from build123d import *

# Parameters (mm, degrees)
SKETCH2_R               = 12.5
BOSS_EXTRUDE1_DEPTH     = 20
CUT_EXTRUDE1_DEPTH      = 13.5
CUT_EXTRUDE1_DEPTH_BACK = 13.5
SKETCH4_R               = 3
CUT_EXTRUDE2_DEPTH      = 3


with BuildPart() as part:
    # Sketch2 → Boss-Extrude1 (new body, symmetric)
    with BuildSketch(Plane(origin=(0, 0, 0), x_dir=(1, 0, 0), z_dir=(0, 1, 0))):
        Circle(SKETCH2_R)
    extrude(amount=BOSS_EXTRUDE1_DEPTH, both=True)

    # Sketch3 → Cut-Extrude1 (cut, two sides)
    with BuildSketch(Plane.XY) as cut_extrude1_sk:
        with BuildLine():
            Line((-7.5, -14), (7.5, -14))
            Line((7.5, -14), (7.5, -12.75))
            ThreePointArc((7.5, -12.75), (7.412263886, -12.186373325), (7.157358145, -11.676083489))
            ThreePointArc((7.157358145, -11.676083489), (3.865958131, -4.691681234), (3.204614294, 3.001030462))
            ThreePointArc((3.204614294, 3.001030462), (4.240621129, 3.863362603), (3.476741803, 4.973954904))
            ThreePointArc((3.476741803, 4.973954904), (3.722208484, 6.12821111), (4.029528967, 7.267559785))
            Line((4.029528967, 7.267559785), (4.622243509, 9.250708497))
            ThreePointArc((4.622243509, 9.250708497), (2.835976896, 9.745509591), (1, 10))
            Line((1, 10), (1, 12))
            Line((1, 12), (2.92625895, 12))
            Line((2.92625895, 12), (2.92625895, 14))
            Line((2.92625895, 14), (1, 14))
            Line((1, 14), (1, 16))
            Line((1, 16), (-1, 16))
            Line((-1, 16), (-1, 14))
            Line((-1, 14), (-2.92625895, 14))
            Line((-2.92625895, 14), (-2.92625895, 12))
            Line((-2.92625895, 12), (-1, 12))
            Line((-1, 12), (-1, 10))
            ThreePointArc((-1, 10), (-2.835976896, 9.745509591), (-4.622243509, 9.250708497))
            Line((-4.622243509, 9.250708497), (-4.029528967, 7.267559785))
            ThreePointArc((-4.029528967, 7.267559785), (-3.722208484, 6.12821111), (-3.476741803, 4.973954904))
            ThreePointArc((-3.476741803, 4.973954904), (-4.240621129, 3.863362603), (-3.204614294, 3.001030462))
            ThreePointArc((-3.204614294, 3.001030462), (-3.865958131, -4.691681234), (-7.157358145, -11.676083489))
            ThreePointArc((-7.157358145, -11.676083489), (-7.412263886, -12.186373325), (-7.5, -12.75))
            Line((-7.5, -12.75), (-7.5, -14))
        make_face()
    extrude(amount=CUT_EXTRUDE1_DEPTH, mode=Mode.SUBTRACT)
    extrude(cut_extrude1_sk.sketch, amount=-CUT_EXTRUDE1_DEPTH_BACK, mode=Mode.SUBTRACT)

    # Sketch4 → Cut-Extrude2 (cut)
    with BuildSketch(Plane(origin=(0, -20, 0), x_dir=(-1, 0, 0), z_dir=(0, -1, 0))):
        Circle(SKETCH4_R)
    extrude(amount=-CUT_EXTRUDE2_DEPTH, mode=Mode.SUBTRACT)


solid = part.part
The listing builds one solid part. Answer for the finished solid, in the listing's coordinates (mm). A direction names the side the tool comes from. Give positions to 0.01 mm unless a question says otherwise; leave off trailing zeros. Order: outer loops, then holes, each group sorted by start corner. A loop starts at its lowest first (then second) coordinate and runs counter-clockwise, first axis right, second up. Notation, with made-up numbers: (-34.75, 16) - (-8.75, 16) arc R3 ccw to (-8.75, 21) - close; hole circle Ø9 at (74.5, 76.25). An arc over 180 degrees is marked (long way). Use one line per item in the form item = value.
1) Consider probe 1 along Z at (x, y) = (0, -19.25); probe 2 along X at (y, z) = (-11, -4). Determine where each line is inside the solid, lowest interval first. Write a range as [from, to].
Verdict:
probe_1 = [-12.5, -3], [3, 12.5]
probe_2 = [-11.84, -6.7], [6.7, 11.84]
2) The mould has two halves that part along X. Classify faces 3 (the flat face through (3, -20, 3)), 4 (the cylindrical face through (-4.243, 3.884, 0.169)): released by +X, released by -X, zero draft, split by the parting line, or undercut.
Verdict:
face_3 = zero draft
face_4 = undercut
3) For faces 1 (the cylindrical face through (3, -19, 0)), 2 (the flat face through (2, 12, 0)), determine the directions among +Z, -Z, +X, -X, +Y, -Y from which every point of the face is accessible in a straight line to the end or side of a thin tool.
Verdict:
face_1 = -Y
face_2 = +Z, -Z
4) Find section A-A on x = 0. Determine the outline of the cut face in (y, z).
Verdict:
outline = (-20, -12.5) - (-14, -12.5) - (-14, 12.5) - (-20, 12.5) - (-20, 3) - (-17, 3) - (-17, -3) - (-20, -3) - close; (16, -12.5) - (20, -12.5) - (20, 12.5) - (16, 12.5) - close
5) Each of these flat-tipped pins is pushed along its axis until it touches: pin 1 (4 mm diameter, centred on x = 2.5, y = 2, fed in from +Z); pin 2 (1.6 mm diameter, centred on y = 15, z = -6, fed in from +X); pin 3 (1 mm diameter, centred on y = -13, z = 4.5, fed in from +X); pin 4 (1 mm diameter, centred on x = 2, z = 2, fed in from -Y). Where does it stop, or does it pass through?
Verdict:
pin_1 = 12.11
pin_2 = 11.37
pin_3 = 11.84
pin_4 = -20
6) Find section D-D on x = -5.5. Determine the outline of the cut face in (y, z).
Verdict:
outline = (-20, -11.22) - (-14, -11.22) - (-14, 11.22) - (-20, 11.22) - close; (-8.94, -11.22) - (20, -11.22) - (20, 11.22) - (-8.94, 11.22) - close
7) Find section C-C on y = 11. Determine the outline of the cut face in (x, z).
Verdict:
outline = (-1, -12.46) - (-1, 12.46) arc R12.5 ccw to start; (1, -12.46) arc R12.5 ccw to (1, 12.46) - close
